Input: part model. Units: mm. Frame: model coordinates. Face numbers are marked on the shaded views. Coordinates: 2 decimals unless noted, no trailing zeros. Write each loop counter-clockwise with the first axis right and the second up, starting at its lowest first coordinate (ties: lowest second). Pieces come first, ordered by that corner, then holes. Notation, with made-up numbers: (88.25, 44) - (145.25, 44) arc R21 cw to (145.25, 66) - close; hole circle Ø11 at (-6.5, 65). An arc over 180 degrees is marked (long way). Use a Markdown table: item, result. Add a question column.
Q1. Section query A-A (z = -2.35). Return the cut outline in (x, y), then the cut area to 3 significant figures.
Q2. Material intervals for probe 1 along Y at (x, z) = (-16, -1.4); probe 2 along Z at (x, y) = (20.5, 25.5), sorted ascending. Write a range as from..to.
Q3. Mould query, pull axis Y, two halves, no side actions, for the marked faces 1 and 2. Classes: released by +Y, released by -Y, zero draft, split by the parting line, or undercut.
Q4. Pin query (flat end, axial travel): P1, Ø1.5, axis at x = 5, y = 1, coming from the -Z side. Return the tip coordinate at first contact, or that it passes through.
Q5. Section query B-B (x = 4.5). Return the cut outline in (y, z), then the cut area to 3 significant figures.
from build123d import *

# Parameters (mm, degrees)
SKETCH1_W           = 56
SKETCH1_H           = 56
BOSS_EXTRUDE1_DEPTH = 2
SKETCH1_3_W         = 56
SKETCH1_3_H         = 56
SKETCH1_3_W_2       = 53
SKETCH1_3_H_2       = 53
BOSS_EXTRUDE2_DEPTH = 3


with BuildPart() as part:
    # Sketch1 → Boss-Extrude1 (new body)
    with BuildSketch(Plane.XY):
        Rectangle(SKETCH1_W, SKETCH1_H)
    extrude(amount=BOSS_EXTRUDE1_DEPTH)

    # Sketch1<3> → Boss-Extrude2 (add)
    with BuildSketch(Plane.XY):
        Rectangle(SKETCH1_3_W, SKETCH1_3_H)
        Rectangle(SKETCH1_3_W_2, SKETCH1_3_H_2, mode=Mode.SUBTRACT)
    extrude(amount=-BOSS_EXTRUDE2_DEPTH)


solid = part.part
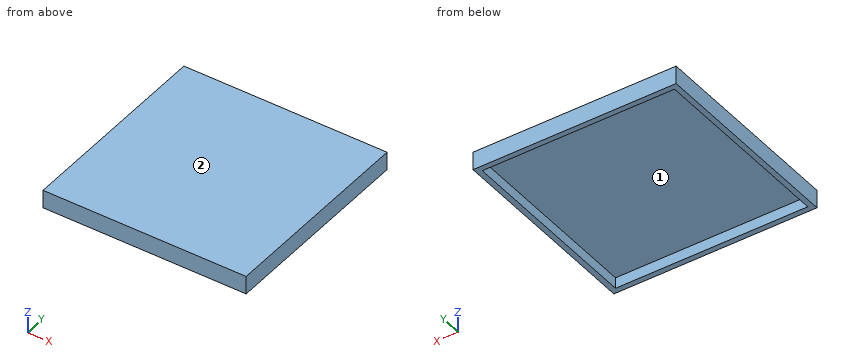
Values follow:
| question | item | result |
|---|---|---|
| 1 | outline | (-28, -28) - (28, -28) - (28, 28) - (-28, 28) - close; hole (-26.5, -26.5) - (26.5, -26.5) - (26.5, 26.5) - (-26.5, 26.5) - close |
| 1 | area | 327 mm2 |
| 2 | probe 1 | -28..-26.5, 26.5..28 |
| 2 | probe 2 | 0..2 |
| 3 | face 1 | undercut |
| 3 | face 2 | zero draft |
| 4 | P1 | z = 0 |
| 5 | outline | (-28, -3) - (-26.5, -3) - (-26.5, 0) - (26.5, 0) - (26.5, -3) - (28, -3) - (28, 2) - (-28, 2) - close |
| 5 | area | 121 mm2 |
